```python
from build123d import *

# Parameters (mm, degrees)
BOSS_EXTRUDE1_DEPTH = 6
SKETCH2_R           = 1.4
CUT_EXTRUDE1_DEPTH  = 30
SKETCH3_R           = 8
CUT_EXTRUDE2_DEPTH  = 3
FILLET1_R           = 10
FILLET2_R           = 10


with BuildPart() as part:
    # Sketch1 → Boss-Extrude1 (new body)
    with BuildSketch(Plane(origin=(0, 0, 0), x_dir=(0, 1, 0), z_dir=(0, 0, 1))):
        with BuildLine():
            Line((6.269968102, 2.5), (9.341687605, 2.5))
            ThreePointArc((9.341687605, 2.5), (11, 3), (12.658312395, 2.5))
            Line((12.658312395, 2.5), (25, 2.5))
            Line((25, 2.5), (25, 6.25))
            Line((25, 6.25), (17, 6.25))
            Line((17, 6.25), (17, 10))
            Line((17, 10), (0, 10))
            ThreePointArc((0, 10), (-10, 0), (0, -10))
            Line((0, -10), (17, -10))
            Line((17, -10), (17, -6.715626424))
            Line((17, -6.715626424), (25, -6.715626424))
            Line((25, -6.715626424), (25, -2.5))
            Line((25, -2.5), (12.658312395, -2.5))
            ThreePointArc((12.658312395, -2.5), (11, -3), (9.341687605, -2.5))
            Line((9.341687605, -2.5), (6.269968102, -2.5))
            ThreePointArc((6.269968102, -2.5), (-6.75, 0), (6.269968102, 2.5))
        make_face()
    extrude(amount=BOSS_EXTRUDE1_DEPTH)

    # Sketch2 → Cut-Extrude1 (cut)
    with BuildSketch(Plane.YZ.offset(10)):
        with Locations(Location((21, 3, 0), (0, 0, 270))):
            Circle(SKETCH2_R)
    extrude(amount=-CUT_EXTRUDE1_DEPTH, mode=Mode.SUBTRACT)

    # Sketch3 → Cut-Extrude2 (cut)
    with BuildSketch(Plane.XY.offset(6)):
        Circle(SKETCH3_R)
    extrude(amount=-CUT_EXTRUDE2_DEPTH, mode=Mode.SUBTRACT)

    # Fillet1
    # the kernel refuses this fillet: 10 mm, written as the material it takes off along each edge
    with BuildSketch(Plane(origin=(10, 17, -18.523694578), x_dir=(-1, 0, 0), z_dir=(0, 0, 1))) as fillet1_piece_1:
        with BuildLine():
            CenterArc((10, 7.409477831), FILLET1_R, 180, 47.812214848)
            Line((0, 7.409477831), (-0.2, 7.409477831))
            Line((-0.2, 7.409477831), (-0.2, 0))
            Line((-0.2, 0), (0, -0.2))
            ThreePointArc((0, -0.2), (1.642186788, -0.2), (3.150061047, -0.148189557))
            Line((3.150061047, -0.148189557), (3.284373576, 0))
        make_face()
    extrude(amount=43.047389155, mode=Mode.SUBTRACT)

    # Fillet2
    # the kernel refuses this fillet: 10 mm, written as the material it takes off along each edge
    with BuildSketch(Plane(origin=(-10, 17, -19.515618745), x_dir=(0, -1, 0), z_dir=(0, 0, 1))) as fillet2_piece_1:
        with BuildLine():
            CenterArc((7.806247498, 10), FILLET2_R, 218.682187453, 51.317812547)
            Line((0, 3.75), (-0.15612495, 3.625))
            ThreePointArc((-0.15612495, 3.625), (-0.2, 1.875), (-0.2, 0))
            Line((-0.2, 0), (0, -0.2))
            Line((0, -0.2), (7.806247498, -0.2))
            Line((7.806247498, -0.2), (7.806247498, 0))
        make_face()
    extrude(amount=45.03123749, mode=Mode.SUBTRACT)


solid = part.part
```
Verification items for the finished model (mm, model axes). A direction names the side the tool comes from. Coordinates: 2 decimals unless noted, no trailing zeros. Loops run counter-clockwise (first coordinate to the right, second up) from the corner with the lowest first, then second, coordinate; pieces in that order, holes last. Notation, with made-up numbers: (86.5, 47.25) - (96.5, 47.25) arc R16 ccw to (96.5, 54.25) - close; hole circle Ø7 at (11.5, 49.25). An arc over 180 degrees is marked (long way). Answer as a JSON object with one key per item and string values.
(1) Cross-section at A-A, the plane y = 8. Record the boundary of the cut face in (x, z), then the cut area to 3 significant figures.
Response:
{"outline": "(-10, 0) - (-2.5, 0) - (-2.5, 6) - (-10, 6) - close; (2.5, 0) - (10, 0) - (10, 6) - (2.5, 6) - close", "area": "90.0 mm²"}
(2) Scan lines: line 1 along X through (y, z) = (8, 0.3); line 2 along Y through (x, z) = (-2.75, 1.3); line 3 along X through (y, z) = (0, 3.65). Record each from-to range of solid material in increasing order.
Response:
{"line 1": "x = -10 to -2.5, 2.5 to 10", "line 2": "y = -9.61 to -6.16, 6.16 to 9.8, 12.2 to 25", "line 3": "x = -10 to -8, 8 to 10"}
(3) Mould release check, pull along X, two halves, no side actions. Record for faces 5 (the cylindrical face through (-3, 11, 3)), 6 (the cylindrical face through (0, -10, 3)), 7 (the flat face through (5, 25, 3)): pulls with the +X half, pulls with the -X half, needs draft (parallel to the pull), parting line crosses it, or undercut.
Response:
{"face 5": "undercut", "face 6": "parting line crosses it", "face 7": "needs draft"}
(4) Cross-section at C-C, the plane y = 21. Record the boundary of the cut face in (x, z), then the cut area to 3 significant figures.
Response:
{"outline": "(-6.25, 0) - (-2.5, 0) - (-2.5, 1.6) - (-6.25, 1.6) - close; (-6.25, 4.4) - (-2.5, 4.4) - (-2.5, 6) - (-6.25, 6) - close; (2.5, 0) - (6.72, 0) - (6.72, 1.6) - (2.5, 1.6) - close; (2.5, 4.4) - (6.72, 4.4) - (6.72, 6) - (2.5, 6) - close", "area": "25.5 mm²"}
(5) Access from +Z, -Z, +X, -X, +Y, -Y to the whole of each face (thin tool, end or side, straight path). Record for faces 1 (the flat face through (-2.5, 8, 2)), 2 (the flat face through (-6.25, 20.2, 1.6)), 3 (the cylindrical face through (3, 11, 3)), 4 (the flat face through (-2, -7, 3)).
Response:
{"face 1": "+Z, -Z, +Y", "face 2": "+Z, -Z, -X, +Y", "face 3": "+Z, -Z", "face 4": "+Z"}
(6) Go/stop test with flat-tipped pins: pin 1 Ø2 at (x, z) = (3.5, 4.5) entering from -Y; pin 2 Ø3 at (y, z) = (20, 4.5) entering from -X; pin 3 Ø1.8 at (y, z) = (20, 2) entering from +X; pin 4 Ø4 at (x, y) = (1.5, 21) entering from +Z. Record where each tip stops, or that it passes through.
Response:
{"pin 1": "stops at y = -9.68", "pin 2": "stops at x = -6.25", "pin 3": "stops at x = 6.72", "pin 4": "stops at z = 6"}
(7) Cross-section at D-D, the plane z = 5.55. Record the boundary of the cut face in (x, y), then the cut area to 3 significant figures.
Response:
{"outline": "(-10, 0) arc R10 ccw to (10, 0) - (10, 9.59) arc R10 ccw to (6.72, 17) - (6.72, 25) - (2.5, 25) - (2.5, 12.66) arc R3 cw to (2.5, 9.34) - (2.5, 7.6) arc R8 cw (long way) to (-2.5, 7.6) - (-2.5, 9.34) arc R3 cw to (-2.5, 12.66) - (-2.5, 25) - (-6.25, 25) - (-6.25, 17) arc R10 ccw to (-10, 9.19) - close", "area": "295 mm²"}
(8) Cross-section at B-B, the plane x = 6.25. Record the boundary of the cut face in (y, z).
Response:
{"outline": "(-7.81, 0) - (-2.55, 0) - (-2.55, 3) - (-4.99, 3) - (-4.99, 6) - (-7.81, 6) - close; (2.55, 0) - (25, 0) - (25, 6) - (4.99, 6) - (4.99, 3) - (2.55, 3) - close; hole circle Ø2.8 at (21, 3)"}
